Design review of the part shown in the three views and the two pictorial views. Dimensions are in mm from the part's minimum x, y and z. Give positions to 0.01 mm unless a question says otherwise; leave off trailing zeros. Order: outer loops, then holes, each group sorted by start corner. A loop starts at its lowest first (then second) coordinate and runs counter-clockwise, first axis right, second up.
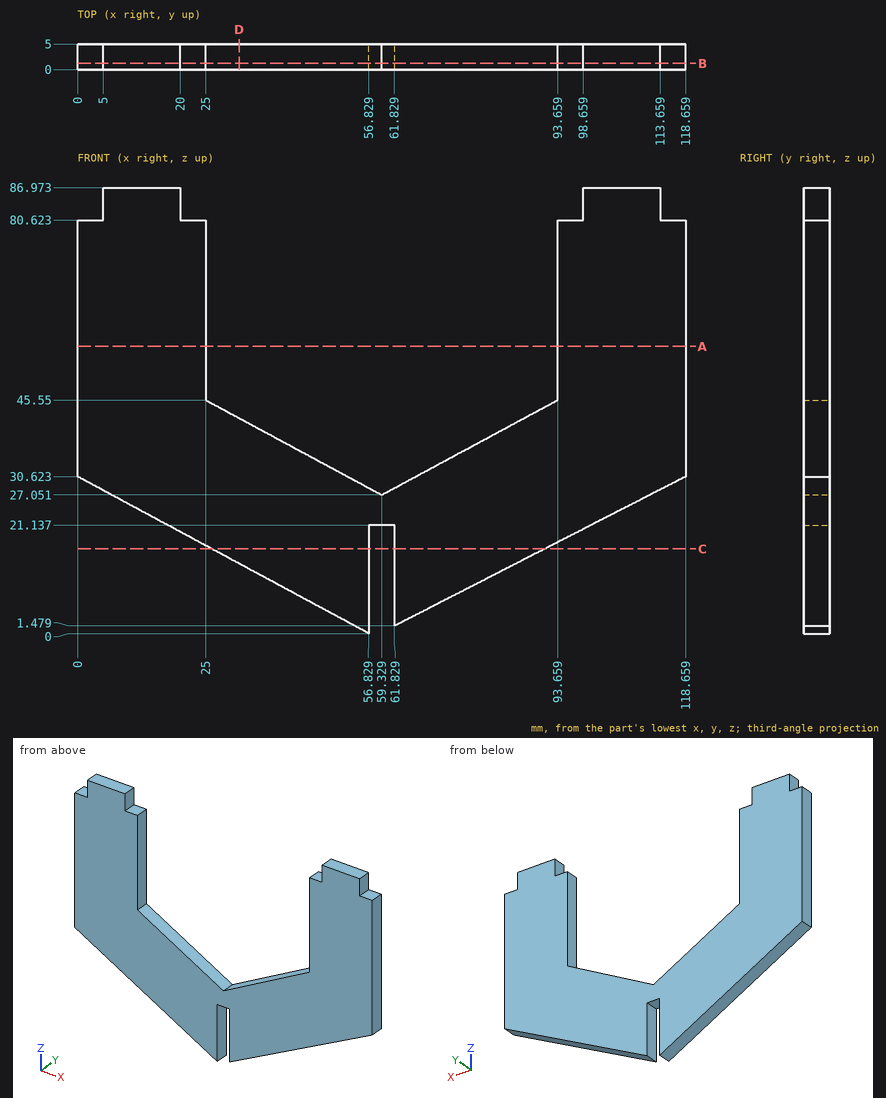
Item 1: Take a section at B-B (y = 1.2). Give the boundary of the cut face in (x, z).
Values found:
outline: (0, 30.62) - (56.83, 0) - (56.83, 21.14) - (61.83, 21.14) - (61.83, 1.48) - (118.66, 30.62) - (118.66, 80.62) - (113.66, 80.62) - (113.66, 86.97) - (98.66, 86.97) - (98.66, 80.62) - (93.66, 80.62) - (93.66, 45.55) - (59.33, 27.05) - (25, 45.55) - (25, 80.62) - (20, 80.62) - (20, 86.97) - (5, 86.97) - (5, 80.62) - (0, 80.62) - close
Item 2: Take a section at D-D (x = 31.5). Give the boundary of the cut face in (y, z), and give its area (3 significant figures).
Values found:
outline: (0, 13.65) - (5, 13.65) - (5, 42.05) - (0, 42.05) - close
area: 142 mm2
Item 3: For line 1 (X direction, y = 3.1, z = 82.5); line 2 (X direction, y = 4.1, z = 64); line 3 (X direction, y = 1.1, z = 22.5) (1 decimal), list the stretches that pass through material, from the lowest coordinate up.
Values found:
line 1: x = 5 to 20, 98.66 to 113.66
line 2: x = 0 to 25, 93.66 to 118.66
line 3: x = 15.1 to 102.8
Item 4: Take a section at A-A (z = 56). Give the boundary of the cut face in (x, y), and give its area (3 significant figures).
Values found:
outline: (0, 0) - (25, 0) - (25, 5) - (0, 5) - close; (93.66, 0) - (118.66, 0) - (118.66, 5) - (93.66, 5) - close
area: 250 mm2
Item 5: Take a section at C-C (z = 16.5). Give the boundary of the cut face in (x, y).
Values found:
outline: (26.21, 0) - (56.83, 0) - (56.83, 5) - (26.21, 5) - close; (61.83, 0) - (91.12, 0) - (91.12, 5) - (61.83, 5) - close
Item 6: Clearance check with flat-ended pins moving along their axes: pin 1 Ø2 at (x, y) = (49, 0.5) entering from -Z; pin 2 Ø2.5 at (x, y) = (115.5, 1.5) entering from +Z; pin 3 Ø1.5 at (x, y) = (59.5, 1.5) entering from -Z. State where each tip first meets the part, or that it passes through.
Values found:
pin 1: stops at z = 3.68
pin 2: stops at z = 80.62
pin 3: stops at z = 21.14
